Could you check a few things on this model? Use its own coordinates, in mm. A direction names the side the tool comes from. Round coordinates to 2 decimals unless told otherwise and drop trailing zeros. Write each loop counter-clockwise with the first axis right and the second up, starting at its lowest first coordinate (ties: lowest second). Pieces come first, ordered by that corner, then holes. Notation, with made-up numbers: (51.5, 65) -> (67.5, 65) arc R23 cw to (67.5, 104) -> close; hole circle Ø8 at (5, 60). An arc over 180 degrees is marked (long way). Answer in a Markdown table with one row per item.
from build123d import *

# Parameters (mm, degrees)
F0_W     = 304.8
F0_H     = 304.8
F1_DEPTH = 711.2
F2_W     = 228.6
F2_H     = 635
F3_DEPTH = 279.4
F4_W     = 228.6
F4_H     = 228.6
F5_DEPTH = 20.32


with BuildPart() as f1:
    # F0 (on Top) → F1 (new body)
    with BuildSketch(Plane.XY):
        with Locations((40.065344, -30.093398)):
            Rectangle(F0_W, F0_H)
    extrude(amount=F1_DEPTH)

    # F2 (on face) → F3 (cut)
    with BuildSketch(Plane.XZ.offset(182.493398)):
        with Locations((40.065344, 355.6)):
            Rectangle(F2_W, F2_H)
    extrude(amount=-F3_DEPTH, mode=Mode.SUBTRACT)

    # F4 (on face) → F5 (cut)
    with BuildSketch(Plane.XY.offset(711.2)):
        with Locations((40.065344, -30.093398)):
            Rectangle(F4_W, F4_H)
    extrude(amount=-F5_DEPTH, mode=Mode.SUBTRACT)


solid = f1.part
1) Imagine slicing it at C-C, the plane x = 10. Please give me the cut outline in (y, z).
Findings:
| item | result |
|---|---|
| outline | (-182.49, 0) -> (122.31, 0) -> (122.31, 711.2) -> (84.21, 711.2) -> (84.21, 690.88) -> (-144.39, 690.88) -> (-144.39, 711.2) -> (-182.49, 711.2) -> (-182.49, 673.1) -> (96.91, 673.1) -> (96.91, 38.1) -> (-182.49, 38.1) -> close |
2) Imagine slicing it at D-D, the plane y = -88. Please give me the cut outline in (x, z).
Findings:
| item | result |
|---|---|
| outline | (-112.33, 0) -> (192.47, 0) -> (192.47, 711.2) -> (154.37, 711.2) -> (154.37, 690.88) -> (-74.23, 690.88) -> (-74.23, 711.2) -> (-112.33, 711.2) -> close; hole (-74.23, 38.1) -> (154.37, 38.1) -> (154.37, 673.1) -> (-74.23, 673.1) -> close |
3) Imagine slicing it at A-A, the plane y = -152. Please give me the cut outline in (x, z), plus the area to 3 significant figures.
Findings:
| item | result |
|---|---|
| outline | (-112.33, 0) -> (192.47, 0) -> (192.47, 711.2) -> (-112.33, 711.2) -> close; hole (-74.23, 38.1) -> (154.37, 38.1) -> (154.37, 673.1) -> (-74.23, 673.1) -> close |
| area | 71,600 mm^2 |
4) Thinking about a two-plate mould opening in Y: for faces 4 (the face through (38, 96.907, 360)), 5 (the face through (154.365, -32, 701)), 6 (the face through (154.365, -45, 351)), which applies, +Y half, -Y half, draft (parallel to the pull), parting line (faces both ways), or undercut?
Findings:
| item | result |
|---|---|
| face 4 | -Y half |
| face 5 | undercut |
| face 6 | draft |
5) For faces 1 (the face through (164, -182.493, 328)), 2 (the face through (38, -45, 38.1)), 3 (the face through (38, 84.207, 701)), which set-ups out of +Z, -Z, +X, -X, +Y, -Y let a thin tool reach every point of the face, with its end or its side?
Findings:
| item | result |
|---|---|
| face 1 | +Z, -Z, +X, -X, -Y |
| face 2 | -Y |
| face 3 | +Z |
6) Imagine slicing it at B-B, the plane z = 615. Please give me the cut outline in (x, y).
Findings:
| item | result |
|---|---|
| outline | (-112.33, -182.49) -> (-74.23, -182.49) -> (-74.23, 96.91) -> (154.37, 96.91) -> (154.37, -182.49) -> (192.47, -182.49) -> (192.47, 122.31) -> (-112.33, 122.31) -> close |
7) For pin 1 (4 mm diameter, centred on x = 151, z = 528, fed in from -Y); pin 2 (1.5 mm diameter, centred on x = -15, y = -133.5, fed in from +Z), each with a flat end and sliding along its axis, tell me the tip position at first contact or that it passes through.
Findings:
| item | result |
|---|---|
| pin 1 | stops at y = 96.91 |
| pin 2 | stops at z = 690.88 |
8) Please list where these lines run through material, in increasing order: line 1 (Z direction, x = 83.5, y = -43); line 2 (X direction, y = -53.5, z = 422); line 3 (Z direction, x = -44, y = -152).
Findings:
| item | result |
|---|---|
| line 1 | z = 0 to 38.1, 673.1 to 690.88 |
| line 2 | x = -112.33 to -74.23, 154.37 to 192.47 |
| line 3 | z = 0 to 38.1, 673.1 to 711.2 |
